Could you check a few things on this model? Use its own coordinates, in mm. A direction names the side the tool comes from. Coordinates: 2 decimals unless noted, no trailing zeros. Loops run counter-clockwise (first coordinate to the right, second up) from the corner with the lowest first, then second, coordinate; pieces in that order, holes last. Notation, with made-up numbers: (-7.75, 13) - (22.25, 13) arc R28 cw to (22.25, 47) - close; hole circle Ø4 at (7, 73). An arc over 180 degrees is marked (long way). One line per item, written item: value. Start each with the question number.
(1) If we section it at A-A on x = -30: Write out the boundary of the cut face in (y, z) (3 decimals).
(2) If we section it at D-D on x = 17: Write out the boundary of the cut face in (y, z) (3 decimals).
(3) If we section it at B-B on y = 2.75: Write out the boundary of the cut face in (x, z).
(4) I'm going to push flat-ended pins straight in: P1, Ø2.5, axis at x = 30, z = 0, coming from the +Y side; P2, Ø13, axis at x = -7.5, z = -1, coming from the +Y side; P3, Ø4, axis at x = 15.5, y = 19, coming from the -Z side; P4, Ø3, axis at x = -39, z = 4.5, coming from the +Y side. Where does each tip first touch, or does it pass through?
(5) On a 3-axis mill with a long thin cutter (end or side, diameter ignored), from which of +Z, -Z, +X, -X, +Y, -Y can I reach the whole of each face in a straight line? I mean faces 4 (the face through (-36.169, 19.423, 4.265)), 5 (the face through (34.86, 4.437, 23.151)), 6 (the face through (-30, 5, 2)), 7 (the face through (36.095, 19.423, 4.371)). Say none if no direction works.
(6) If I drill on line 1 along X through (y, z) = (16.75, 0) (3 decimals); line 2 along X through (y, z) = (2.75, 0); line 3 along Z through (x, y) = (-8, 21.75), over which ranges is the centre line in solid material (lowest first)? Write a range as from..to.
(7) If we mould it in two halves opening along Z, with no side actions, what happens to faces 1 (the face through (29, 12, -10)), 2 (the face through (15.5, 21.97, 23.15)), 3 (the face through (0, 2, 10))? For each: pulls with the +Z half, pulls with the -Z half, needs draft (parallel to the pull), parting line crosses it, or undercut.
(8) If we section it at C-C on z = 23: Write out the boundary of the cut face in (x, y), then the cut area to 3 significant figures.
```python
from build123d import *

# Parameters (mm, degrees)
SKETCH1_R               = 2.51
BOSS_EXTRUDE1_DEPTH     = 5
SKETCH2_R               = 6.125
SKETCH2_R_2             = 4.125
BOSS_EXTRUDE2_DEPTH     = 20
SKETCH1_3_W             = 20
SKETCH1_3_H             = 15
BOSS_EXTRUDE3_DEPTH     = 25
SKETCH3_W               = 17.5
SKETCH3_H               = 6.5
CUT_EXTRUDE2_DEPTH      = 21.5
CUT_EXTRUDE3_REACH      = 64.249
SKETCH4_R               = 2.05
SKETCH5_W               = 13.25
SKETCH5_H               = 9
CUT_EXTRUDE4_DEPTH      = 97.695397829
BOSS_EXTRUDE4_DEPTH     = 90
SKETCH9_R               = 1.5
CUT_EXTRUDE6_DEPTH      = 56.226804735
BOSS_EXTRUDE9_OUTLINE_W = 26.5
BOSS_EXTRUDE9_OUTLINE_H = 20
BOSS_EXTRUDE9_OUTLINE_R = 6.125
BOSS_EXTRUDE9_DEPTH     = 9
SKETCH12_R              = 7.5
SKETCH12_R_2            = 6.125
SKETCH12_W              = 5
SKETCH12_H              = 0.387499923
BOSS_EXTRUDE10_DEPTH    = 11
BOSS_EXTRUDE11_START    = -25
SKETCH13_W              = 50
SKETCH13_H              = 3.75
BOSS_EXTRUDE11_DEPTH    = 25
BOSS_EXTRUDE12_DEPTH    = 9
BOSS_EXTRUDE13_DEPTH    = 3.75
SKETCH16_R              = 1.55
SKETCH16_R_2            = 1.5
CUT_EXTRUDE7_DEPTH      = 38


# Read off the part's stored shape, not the designer's step: Boss-Extrude9
with BuildPart() as part:
    # Sketch1 → Boss-Extrude1 (new body)
    with BuildSketch(Plane(origin=(0, 0, 0), x_dir=(1, 0, 0), z_dir=(0, 1, 0))):
        with BuildLine():
            ThreePointArc((-2.51, -9.999999226), (0, -7.489999226), (2.51, -9.999999226))
            Line((2.51, -9.999999226), (45, -9.999999226))
            Line((45, -9.999999226), (45, 10.000000774))
            Line((45, 10.000000774), (2.51, 10.000000774))
            ThreePointArc((2.51, 10.000000774), (0, 7.490000774), (-2.51, 10.000000774))
            Line((-2.51, 10.000000774), (-45, 10.000000774))
            Line((-45, 10.000000774), (-45, -9.999999226))
            Line((-45, -9.999999226), (-2.51, -9.999999226))
        make_face()
        with BuildLine():
            ThreePointArc((-7.500032569, 0.22419454), (-10, -2.509999226), (-12.499967431, 0.22419454))
            ThreePointArc((-12.499967431, 0.22419454), (-10, 2.510000774), (-7.500032569, 0.22419454))
        make_face(mode=Mode.SUBTRACT)
        with BuildLine():
            ThreePointArc((2.499967431, 0.22419454), (0, -2.509999226), (-2.499967431, 0.22419454))
            ThreePointArc((-2.499967431, 0.22419454), (0, 2.510000774), (2.499967431, 0.22419454))
        make_face(mode=Mode.SUBTRACT)
        with Locations(Location((10, 7.74e-07, 0), (0, 0, 270))):
            Circle(SKETCH1_R, mode=Mode.SUBTRACT)
    extrude(amount=BOSS_EXTRUDE1_DEPTH)

    # Sketch2 → Boss-Extrude2 (add)
    # profile 1 of 2: a face of its own
    with BuildSketch(Plane(origin=(0, 5, 0), x_dir=(1, 0, 0), z_dir=(0, 1, 0))):
        with Locations(Location((-30, 0, 0), (0, 0, 270))):
            Circle(SKETCH2_R)
        with Locations(Location((-30, 0, 0), (0, 0, 270))):
            Circle(SKETCH2_R_2, mode=Mode.SUBTRACT)
    # profile 2 of 2: a face of its own
    with BuildSketch(Plane(origin=(0, 5, 0), x_dir=(1, 0, 0), z_dir=(0, 1, 0))):
        with Locations(Location((30, 0, 0), (0, 0, 270))):
            Circle(SKETCH2_R)
        with Locations(Location((30, 0, 0), (0, 0, 270))):
            Circle(SKETCH2_R_2, mode=Mode.SUBTRACT)
    extrude(amount=BOSS_EXTRUDE2_DEPTH)

    # Sketch1<3> → Boss-Extrude3 (add)
    with BuildSketch(Plane(origin=(0, 0, 0), x_dir=(1, 0, 0), z_dir=(0, 1, 0))):
        with Locations((35, -17.499999226)):
            Rectangle(SKETCH1_3_W, SKETCH1_3_H)
        with Locations((-35, -17.499999226)):
            Rectangle(SKETCH1_3_W, SKETCH1_3_H)
    extrude(amount=BOSS_EXTRUDE3_DEPTH)

    # Sketch3 → Cut-Extrude2 (cut)
    with BuildSketch(Plane(origin=(0, 25, 0), x_dir=(1, 0, 0), z_dir=(0, 1, 0))):
        with Locations((36.25, -17.999999226)):
            Rectangle(SKETCH3_W, SKETCH3_H)
        with Locations((-36.25, -17.999999226)):
            Rectangle(SKETCH3_W, SKETCH3_H)
    extrude(amount=-CUT_EXTRUDE2_DEPTH, mode=Mode.SUBTRACT)

    # Cut-Extrude3: up to this face of the body (flat: up to its plane)
    cut_extrude3_end = Plane(part.part.faces().sort_by_distance((35, 15, 9.999999226))[0])
    # Sketch4 → Cut-Extrude3 (cut, up to the picked face)
    with BuildSketch(Plane.XY.offset(24.999999226), mode=Mode.PRIVATE) as cut_extrude3_sk1:
        with Locations((37.5, 20.5)):
            Circle(SKETCH4_R)
    cut_extrude3_tool1 = split(extrude(cut_extrude3_sk1.sketch, amount=-CUT_EXTRUDE3_REACH, mode=Mode.PRIVATE), bisect_by=cut_extrude3_end, keep=Keep.BOTH, mode=Mode.PRIVATE)
    # Sketch4 → Cut-Extrude3 (cut, up to the picked face)
    with BuildSketch(Plane.XY.offset(24.999999226), mode=Mode.PRIVATE) as cut_extrude3_sk2:
        with Locations((-37.5, 20.5)):
            Circle(SKETCH4_R)
    cut_extrude3_tool2 = split(extrude(cut_extrude3_sk2.sketch, amount=-CUT_EXTRUDE3_REACH, mode=Mode.PRIVATE), bisect_by=cut_extrude3_end, keep=Keep.BOTH, mode=Mode.PRIVATE)
    add(cut_extrude3_tool1.solids().sort_by(Axis((37.5, 20.5, 24.999999), (0, 0, -1)))[0], mode=Mode.SUBTRACT)
    add(cut_extrude3_tool2.solids().sort_by(Axis((-37.5, 20.5, 24.999999), (0, 0, -1)))[0], mode=Mode.SUBTRACT)

    # Sketch5 → Cut-Extrude4 (cut, through all)
    with BuildSketch(Plane(origin=(45, 0, 0), x_dir=(0, 0, -1), z_dir=(1, 0, 0))):
        with Locations((-18.374999226, 4.5)):
            Rectangle(SKETCH5_W, SKETCH5_H)
    extrude(amount=-CUT_EXTRUDE4_DEPTH, mode=Mode.SUBTRACT)

    # Sketch6 → Boss-Extrude4 (add, through all)
    with BuildSketch(Plane(origin=(45, 0, 0), x_dir=(0, 0, -1), z_dir=(1, 0, 0))):
        Polygon((-9.999999226, 15), (-6.125, 5), (-9.999999226, 5), align=None)
    extrude(amount=-BOSS_EXTRUDE4_DEPTH)

    # Sketch9 → Cut-Extrude6 (cut, through all)
    with BuildSketch(Plane(origin=(0, 5, 0), x_dir=(1, 0, 0), z_dir=(0, 1, 0))):
        with Locations(Location((30, 0, 0), (0, 0, 270))):
            Circle(SKETCH9_R)
        with Locations(Location((-30, 0, 0), (0, 0, 270))):
            Circle(SKETCH9_R)
    extrude(amount=-CUT_EXTRUDE6_DEPTH, mode=Mode.SUBTRACT)

    # Boss-Extrude9 outline → Boss-Extrude9 (add)
    # profile 1 of 2: a face of its own
    with BuildSketch(Plane(origin=(0, 5, 0), x_dir=(1, 0, 0), z_dir=(0, 1, 0))):
        with Locations((-31.75, 7.74e-07)):
            Rectangle(BOSS_EXTRUDE9_OUTLINE_W, BOSS_EXTRUDE9_OUTLINE_H)
        with Locations((-30, 0)):
            Circle(BOSS_EXTRUDE9_OUTLINE_R, mode=Mode.SUBTRACT)
    # profile 2 of 2: a face of its own
    with BuildSketch(Plane(origin=(0, 5, 0), x_dir=(1, 0, 0), z_dir=(0, 1, 0))):
        with Locations((31.75, 7.74e-07)):
            Rectangle(BOSS_EXTRUDE9_OUTLINE_W, BOSS_EXTRUDE9_OUTLINE_H)
        with Locations((30, 0)):
            Circle(BOSS_EXTRUDE9_OUTLINE_R, mode=Mode.SUBTRACT)
    extrude(amount=BOSS_EXTRUDE9_DEPTH)

    # Sketch12 → Boss-Extrude10 (add)
    # profile 1 of 8: a face of its own
    with BuildSketch(Plane(origin=(0, 14, 0), x_dir=(1, 0, 0), z_dir=(0, 1, 0))):
        with BuildLine():
            Line((32.5, -9.612499303), (32.5, -7.071067812))
            ThreePointArc((32.5, -7.071067812), (30, -7.5), (27.5, -7.071067812))
            Line((27.5, -7.071067812), (27.5, -9.612499303))
            Line((27.5, -9.612499303), (32.5, -9.612499303))
        make_face()
    # profile 2 of 8: a face of its own
    with BuildSketch(Plane(origin=(0, 14, 0), x_dir=(1, 0, 0), z_dir=(0, 1, 0))):
        with Locations((30, 0)):
            Circle(SKETCH12_R)
        with Locations((30, 0)):
            Circle(SKETCH12_R_2, mode=Mode.SUBTRACT)
    # profile 3 of 8: a face of its own
    with BuildSketch(Plane(origin=(0, 14, 0), x_dir=(1, 0, 0), z_dir=(0, 1, 0))):
        with BuildLine():
            Line((-32.5, -7.071067812), (-32.5, -9.999999226))
            Line((-32.5, -9.999999226), (-27.5, -9.999999226))
            Line((-27.5, -9.999999226), (-27.5, -7.071067812))
            ThreePointArc((-27.5, -7.071067812), (-30, -7.5), (-32.5, -7.071067812))
        make_face()
    # profile 4 of 8: a face of its own
    with BuildSketch(Plane(origin=(0, 14, 0), x_dir=(1, 0, 0), z_dir=(0, 1, 0))):
        with Locations((-30, 0)):
            Circle(SKETCH12_R)
        with Locations((-30, 0)):
            Circle(SKETCH12_R_2, mode=Mode.SUBTRACT)
    # profile 5 of 8: a face of its own
    with BuildSketch(Plane(origin=(0, 14, 0), x_dir=(1, 0, 0), z_dir=(0, 1, 0))):
        with Locations((30, -9.806249264)):
            Rectangle(SKETCH12_W, SKETCH12_H)
    # profile 6 of 8: a face of its own
    with BuildSketch(Plane(origin=(0, 14, 0), x_dir=(1, 0, 0), z_dir=(0, 1, 0))):
        with BuildLine():
            Line((27.5, -9.612499303), (27.5, -7.071067812))
            ThreePointArc((27.5, -7.071067812), (25.657627479, 6.115047088), (37.499939934, 0.030016408))
            Line((37.499939934, 0.030016408), (45, 0.193750736))
            Line((45, 0.193750736), (45, 10.000000774))
            Line((45, 10.000000774), (18.5, 10.000000774))
            Line((18.5, 10.000000774), (18.5, -9.612499303))
            Line((18.5, -9.612499303), (27.5, -9.612499303))
        make_face()
    # profile 7 of 8: a face of its own
    with BuildSketch(Plane(origin=(0, 14, 0), x_dir=(1, 0, 0), z_dir=(0, 1, 0))):
        with BuildLine():
            Line((-27.5, -7.071067812), (-27.5, -9.999999226))
            Line((-27.5, -9.999999226), (-25, -9.999999226))
            Line((-25, -9.999999226), (-18.5, -9.999999226))
            Line((-18.5, -9.999999226), (-18.5, -9.612499303))
            Line((-18.5, -9.612499303), (-18.5, 10.000000774))
            Line((-18.5, 10.000000774), (-45, 10.000000774))
            Line((-45, 10.000000774), (-45, 0.193750736))
            Line((-45, 0.193750736), (-37.499939934, 0.030016408))
            ThreePointArc((-37.499939934, 0.030016408), (-29.984991766, 7.499984984), (-22.5, 0))
            ThreePointArc((-22.5, 0), (-23.876275643, -4.330127019), (-27.5, -7.071067812))
        make_face()
    # profile 8 of 8: a face of its own
    with BuildSketch(Plane(origin=(0, 14, 0), x_dir=(1, 0, 0), z_dir=(0, 1, 0))):
        Polygon((27.5, -9.999999226), (27.5, -9.612499303), (18.5, -9.612499303), (18.5, -9.999999226), (25, -9.999999226), align=None)
    extrude(amount=BOSS_EXTRUDE10_DEPTH)

    # Sketch13 → Boss-Extrude11 (add)
    with BuildSketch(Plane(origin=(0, 25, 0), x_dir=(1, 0, 0), z_dir=(0, 1, 0)).offset(BOSS_EXTRUDE11_START)):
        with Locations((0, -23.124999226)):
            Rectangle(SKETCH13_W, SKETCH13_H)
        Polygon((25, -12.749999226), (25, -9.999999226), (18.5, -9.999999226), (-25, -9.999999226), (-25, -12.749999226), align=None)
    extrude(amount=BOSS_EXTRUDE11_DEPTH)

    # Sketch14 → Boss-Extrude12 (add)
    with BuildSketch(Plane.XZ.offset(-9)):
        Polygon((-25, 14.749999226), (-27.5, 14.749999226), (-45, 14.749999226), (-45, 11.749999226), (-25, 11.749999226), (-25, 12.749999226), align=None)
        Polygon((45, 14.749999226), (27.5, 14.749999226), (25, 14.749999226), (25, 12.749999226), (25, 11.749999226), (45, 11.749999226), align=None)
    extrude(amount=BOSS_EXTRUDE12_DEPTH)

    # Sketch15 → Boss-Extrude13 (add)
    with BuildSketch(Plane.XY.offset(24.999999226)):
        Polygon((-45, 9), (-25, 0), (-25, 9), align=None)
        Polygon((25, 0), (45, 9), (25, 9), align=None)
    extrude(amount=-BOSS_EXTRUDE13_DEPTH)

    # Sketch16 → Cut-Extrude7 (cut)
    with BuildSketch(Plane.XY.offset(24.999999226)):
        with Locations((-1.99973684, 22)):
            Circle(SKETCH16_R)
        with Locations((17, 21.9)):
            Circle(SKETCH16_R_2)
    extrude(amount=-CUT_EXTRUDE7_DEPTH, mode=Mode.SUBTRACT)


solid = part.part
```
Values:
1. outline: (0, -10) - (25, -10) - (25, -4.125) - (5, -4.125) - (5, -1.5) - (0, -1.5) - close; (0, 1.5) - (5, 1.5) - (5, 4.125) - (25, 4.125) - (25, 14.75) - (0, 14.75) - close; (2.25, 21.25) - (25, 21.25) - (25, 25) - (2.25, 25) - close
2. outline: (0, -10) - (5, -10) - (5, 6.125) - (15, 10) - (20.4, 10) - (20.4, 12.75) - (0, 12.75) - close; (0, 21.25) - (20.4, 21.25) - (20.4, 25) - (0, 25) - close; (23.4, 10) - (25, 10) - (25, 12.75) - (23.4, 12.75) - close; (23.4, 21.25) - (25, 21.25) - (25, 25) - (23.4, 25) - close
3. outline: (-45, -10) - (-2.51, -10) arc R2.51 cw to (2.51, -10) - (45, -10) - (45, 14.75) - (25, 14.75) - (25, 12.75) - (-25, 12.75) - (-25, 14.75) - (-45, 14.75) - close; (-31.11, 21.25) - (31.11, 21.25) - (31.11, 25) - (-31.11, 25) - close; hole circle Ø3 at (-30, 0); hole circle Ø5.02 at (-10, 0); hole circle Ø5.02 at (0, 0); hole (-2.51, 10) arc R2.51 ccw to (2.51, 10) - close; hole circle Ø5.02 at (10, 0); hole circle Ø3 at (30, 0)
4. P1: passes through
4. P2: stops at y = 5
4. P3: stops at z = 10
4. P4: stops at y = 14
5. face 4: -X, +Y
5. face 5: +Z, +X, -Y
5. face 6: +Y
5. face 7: +X, +Y
6. line 1: x = -37.5..-34.125, -25.875..-18.5, 18.5..25.875, 34.125..37.5
6. line 2: x = -45..-31.5, -28.5..-12.51, -7.49..-2.51, 2.51..7.49, 12.51..28.5, 31.5..45
6. line 3: z = 10..12.75, 21.25..25
7. face 1: pulls with the -Z half
7. face 2: needs draft
7. face 3: undercut
8. outline: (-45, 9) - (-25, 0) - (25, 0) - (45, 9) - (45, 25) - (-45, 25) - close; hole circle Ø4.1 at (-37.5, 20.5); hole circle Ø3.1 at (-2, 22); hole circle Ø3 at (17, 21.9); hole circle Ø4.1 at (37.5, 20.5)
8. area: 2,030 mm2
